from build123d import *

# Parameters (mm, degrees)
F0_R     = 12.7
F1_DEPTH = 50.8
F2_R     = 12.7


with BuildPart() as f1:
    # F0 (on Front) → F1 (new body)
    with BuildSketch(Plane.XZ):
        with BuildLine():
            ThreePointArc((174.6427991592, -2.9811911121), (174.7023389384, 0.1935607732), (174.7221865654, 3.3688088879))
            ThreePointArc((174.7221865654, 3.3688088879), (174.7023389185, 6.5440585944), (174.6427990796, 9.7188120708))
            ThreePointArc((174.6427990796, 9.7188120708), (155.3875872141, 100.5704021794), (104.761301674, 178.4276678755))
            ThreePointArc((104.761301674, 178.4276678755), (100.3273078611, 182.973932435), (95.781043246, 187.4079261909))
            ThreePointArc((95.781043246, 187.4079261909), (17.9237769154, 238.034210755), (-72.9278134346, 257.2894214817))
            ThreePointArc((-72.9278134346, 257.2894214817), (-79.2778150265, 257.3688088879), (-85.6278166175, 257.2894214021))
            ThreePointArc((-85.6278166175, 257.2894214021), (-176.4794067261, 238.0342095366), (-254.3366724222, 187.4079239965))
            ThreePointArc((-254.3366724222, 187.4079239965), (-258.8829369817, 182.9739301836), (-263.3169307376, 178.4276655685))
            ThreePointArc((-263.3169307376, 178.4276655685), (-313.9432153017, 100.5703992379), (-333.1984260284, 9.7188088879))
            ThreePointArc((-333.1984260284, 9.7188088879), (-333.2778134346, 3.368807296), (-333.1984259488, -2.981194295))
            ThreePointArc((-333.1984259488, -2.981194295), (-313.9432140833, -93.8327844036), (-263.3169285432, -171.6900500997))
            ThreePointArc((-263.3169285432, -171.6900500997), (-258.8829347303, -176.2363146592), (-254.3366701152, -180.6703084151))
            ThreePointArc((-254.3366701152, -180.6703084151), (-176.4794037846, -231.2965929792), (-85.6278134346, -250.5518037059))
            ThreePointArc((-85.6278134346, -250.5518037059), (-79.2778118427, -250.6311911121), (-72.9278102517, -250.5518036263))
            ThreePointArc((-72.9278102517, -250.5518036263), (17.9237798569, -231.2965917608), (95.781045553, -180.6703062207))
            ThreePointArc((95.781045553, -180.6703062207), (100.3273101125, -176.2363124078), (104.7613038684, -171.6900477927))
            ThreePointArc((104.7613038684, -171.6900477927), (155.3875884325, -93.8327814621), (174.6427991592, -2.9811911121))
        make_face()
        with BuildLine():
            Line((-218.4016056024, -144.7352439022), (-96.7847279201, -23.11836622))
            ThreePointArc((-96.7847279201, -23.11836622), (-91.4280109116, -25.9643668909), (-85.6278134346, -27.7397108454))
            Line((-85.6278134346, -27.7397108454), (-85.6278134346, -199.7319481269))
            ThreePointArc((-85.6278134346, -199.7319481269), (-157.0390854202, -184.3635127277), (-218.4016056024, -144.7352439022))
        make_face(mode=Mode.SUBTRACT)
        with BuildLine():
            ThreePointArc((-227.3818640444, -135.7549856009), (-267.0101338316, -74.3924660397), (-282.3785703499, -2.981194295))
            Line((-282.3785703499, -2.981194295), (-110.3863325182, -2.981194295))
            ThreePointArc((-110.3863325182, -2.981194295), (-108.6109879703, -8.7813915903), (-105.7649867513, -14.1381083077))
            Line((-105.7649867513, -14.1381083077), (-227.3818640444, -135.7549856009))
        make_face(mode=Mode.SUBTRACT)
        with BuildLine():
            Line((-72.9278102517, -199.7319480274), (-72.9278102517, -27.7397101957))
            ThreePointArc((-72.9278102517, -27.7397101957), (-67.1276129564, -25.9643656478), (-61.770896239, -23.1183644288))
            Line((-61.770896239, -23.1183644288), (59.8459810542, -144.7352417219))
            ThreePointArc((59.8459810542, -144.7352417219), (-1.516538507, -184.3635115091), (-72.9278102517, -199.7319480274))
        make_face(mode=Mode.SUBTRACT)
        with BuildLine():
            Line((68.8262393555, -135.7549832799), (-52.7906383267, -14.1381055976))
            ThreePointArc((-52.7906383267, -14.1381055976), (-49.9446376558, -8.7813885891), (-48.1692937013, -2.9811911121))
            Line((-48.1692937013, -2.9811911121), (123.8229435802, -2.9811911121))
            ThreePointArc((123.8229435802, -2.9811911121), (108.454508181, -74.3924630977), (68.8262393555, -135.7549832799))
        make_face(mode=Mode.SUBTRACT)
        with BuildLine():
            Line((-227.3818662247, 142.4926010557), (-105.7649885425, 20.8757233734))
            ThreePointArc((-105.7649885425, 20.8757233734), (-108.6109892134, 15.5190063649), (-110.3863331679, 9.7188088879))
            Line((-110.3863331679, 9.7188088879), (-282.3785704494, 9.7188088879))
            ThreePointArc((-282.3785704494, 9.7188088879), (-267.0101350502, 81.1300808735), (-227.3818662247, 142.4926010557))
        make_face(mode=Mode.SUBTRACT)
        with BuildLine():
            Line((-85.6278166175, 206.4695658032), (-85.6278166175, 34.4773279715))
            ThreePointArc((-85.6278166175, 34.4773279715), (-91.4280139128, 32.7019834236), (-96.7847306302, 29.8559822046))
            Line((-96.7847306302, 29.8559822046), (-218.4016079234, 151.4728594977))
            ThreePointArc((-218.4016079234, 151.4728594977), (-157.0390883622, 191.1011292849), (-85.6278166175, 206.4695658032))
        make_face(mode=Mode.SUBTRACT)
        with Locations((-79.2778134346, 3.3688088879)):
            Circle(F0_R, mode=Mode.SUBTRACT)
        with BuildLine():
            Line((123.8229434807, 9.7188120708), (-48.169294351, 9.7188120708))
            ThreePointArc((-48.169294351, 9.7188120708), (-49.9446388989, 15.5190093661), (-52.7906401179, 20.8757260835))
            Line((-52.7906401179, 20.8757260835), (68.8262371752, 142.4926033767))
            ThreePointArc((68.8262371752, 142.4926033767), (108.4545069624, 81.1300838155), (123.8229434807, 9.7188120708))
        make_face(mode=Mode.SUBTRACT)
        with BuildLine():
            ThreePointArc((-61.7708989491, 29.8559839958), (-67.1276159576, 32.7019846667), (-72.9278134346, 34.4773286212))
            Line((-72.9278134346, 34.4773286212), (-72.9278134346, 206.4695659027))
            ThreePointArc((-72.9278134346, 206.4695659027), (-1.516541449, 191.1011305035), (59.8459787332, 151.472861678))
            Line((59.8459787332, 151.472861678), (-61.7708989491, 29.8559839958))
        make_face(mode=Mode.SUBTRACT)
    extrude(amount=F1_DEPTH)

    # F2
    f2_edges = [f1.edges().sort_by_distance(p)[0] for p in [
        (-254.33667, -50.8, -180.670308),
        (-254.33667, 0, -180.670308),
    ]]
    fillet(f2_edges, radius=F2_R)


solid = f1.part
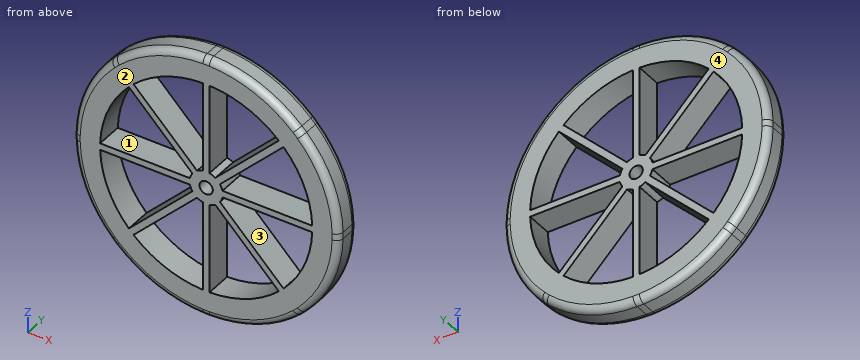
Check sheet for the modelled part. Datum: model origin and axes. Units: mm. Face numbers are marked on the shaded views. A direction names the side the tool comes from. Round coordinates to 2 decimals unless told otherwise and drop trailing zeros.
1. Set-up check for the marked faces 1 and 2: record each of +Z, -Z, +X, -X, +Y, -Y from which the full face is reachable in a straight line by a thin tool's end or side.
2. Sectioned sample at A-A on x = -198. Give the number of separate pieces and of enclosed holes in the cut face, and give its area (3 significant figures).
3. Scan lines: probe 1 along X at (y, z) = (-36.5, 73.5); probe 2 along X at (y, z) = (-6, -171); probe 3 along X at (y, z) = (-21.5, 98.5). Record each from-to range of solid material in increasing order.
4. Mould release check, pull along X, two halves, no side actions. Record for the marked faces 3 and 4: released by +X, released by -X, zero draft, split by the parting line, or undercut.
5. Gauge pin test, flat ends, axial feed: pin 1 Ø1 at (x, y) = (-35, -25) entering from -Z; pin 2 Ø3 at (x, y) = (-202.5, -12) entering from +Z; pin 3 Ø8 at (x, y) = (-215, -6) entering from +Z; pin 4 Ø5 at (x, z) = (24.5, 97) entering from -Y. Record the tip position at first contact, or that the pin passes through.
Recorded:
1. face 1: +Y, -Y
1. face 2: +Z, -Z, +X, -X, -Y
2. separate pieces: 5
2. enclosed holes: 0
2. area: 8,370 mm2
3. probe 1: x = -323.4 to -269.99, -158.39 to -140.43, -85.63 to -72.93, -18.13 to -0.17, 111.44 to 164.85
3. probe 2: x = -261.33 to -183.61, -85.63 to -72.93, 25.06 to 102.78
3. probe 3: x = -314.79 to -258.83, -183.39 to -165.43, -85.63 to -72.93, 6.87 to 24.83, 100.28 to 156.23
4. face 3: undercut
4. face 4: zero draft
5. pin 1: stops at z = -246.83
5. pin 2: stops at z = 226.29
5. pin 3: stops at z = 219.18
5. pin 4: stops at y = -50.8
